The model under review builds one solid part; all positions refer to its coordinate system, in mm. Coordinates: 2 decimals unless noted, no trailing zeros. Order: outer loops, then holes, each group sorted by start corner. A loop starts at its lowest first (then second) coordinate and runs counter-clockwise, first axis right, second up.
from build123d import *

# Parameters (mm, degrees)
SKETCH_1_R      = 1.5
SKETCH_1_R_2    = 20
SKETCH_1_R_3    = 2.1
SKETCH_1_R_4    = 2
SKETCH_1_W      = 8.4
SKETCH_1_H      = 4.4
EXTRUDE_1_DEPTH = 4
EXTRUDE_2_DEPTH = 4
EXTRUDE_4_DEPTH = 4


with BuildPart() as part:
    # 草图1 → 凸台-拉伸1 (new body)
    with BuildSketch(Plane.XY):
        with BuildLine():
            Line((7.027428163, -5.002489357), (18.190287148, -14.686974418))
            ThreePointArc((18.190287148, -14.686974418), (47.018030055, -25.451404949), (75.84881126, -14.695114654))
            Line((75.84881126, -14.695114654), (87.027428163, -5.002489357))
            Line((87.027428163, -5.002489357), (87.027428163, 75.054738201))
            Line((87.027428163, 75.054738201), (21.027428163, 141.054738201))
            Line((21.027428163, 141.054738201), (-114.887663771, 141.054738201))
            ThreePointArc((-114.887663771, 141.054738201), (-124.126459096, 134.881572525), (-121.958731583, 123.983670389))
            Line((-121.958731583, 123.983670389), (-90.203942848, 92.228881654))
            Line((-90.203942848, 92.228881654), (7.027428163, -5.002489357))
        make_face()
        with Locations((-52.972571837, 135.054738201)):
            Circle(SKETCH_1_R, mode=Mode.SUBTRACT)
        with Locations((47.027428163, 15.054738201)):
            Circle(SKETCH_1_R_2, mode=Mode.SUBTRACT)
        with Locations(Location((-22.972571837, 135.054738201, 0), (0, 0, 180))):
            Circle(SKETCH_1_R, mode=Mode.SUBTRACT)
        with Locations((7.027428163, 135.054738201)):
            Circle(SKETCH_1_R, mode=Mode.SUBTRACT)
        with Locations(Location((-112.972571837, 135.054738201, 0), (0, 0, 180))):
            Circle(SKETCH_1_R, mode=Mode.SUBTRACT)
        with Locations((-82.972571837, 135.054738201)):
            Circle(SKETCH_1_R, mode=Mode.SUBTRACT)
        with Locations((49.784787476, 103.812097514)):
            Circle(SKETCH_1_R, mode=Mode.SUBTRACT)
        with Locations(Location((70.997990912, 82.598894078, 0), (0, 0, 180))):
            Circle(SKETCH_1_R, mode=Mode.SUBTRACT)
        with Locations(Location((28.571584041, 125.025300949, 0), (0, 0, 180))):
            Circle(SKETCH_1_R, mode=Mode.SUBTRACT)
        with Locations((70.597428163, 38.624738201)):
            Circle(SKETCH_1_R_3, mode=Mode.SUBTRACT)
        with Locations((70.597428163, -8.515261799)):
            Circle(SKETCH_1_R_3, mode=Mode.SUBTRACT)
        with Locations((23.457428163, -8.515261799)):
            Circle(SKETCH_1_R_3, mode=Mode.SUBTRACT)
        with Locations((23.457428163, 38.624738201)):
            Circle(SKETCH_1_R_3, mode=Mode.SUBTRACT)
        with Locations((-83.04451802, 93.554738201)):
            Circle(SKETCH_1_R, mode=Mode.SUBTRACT)
        with Locations((-61.831314585, 72.341534765)):
            Circle(SKETCH_1_R, mode=Mode.SUBTRACT)
        with Locations(Location((-104.257721456, 114.767941637, 0), (0, 0, 180))):
            Circle(SKETCH_1_R, mode=Mode.SUBTRACT)
        with Locations((20.166275086, 57.226748532)):
            Circle(SKETCH_1_R_4, mode=Mode.SUBTRACT)
        with Locations((-6.694877991, 99.398758863)):
            Circle(SKETCH_1_R_4, mode=Mode.SUBTRACT)
        with Locations((-37.972571837, 135.054738201)):
            Rectangle(SKETCH_1_W, SKETCH_1_H, mode=Mode.SUBTRACT)
        with Locations((-7.972571837, 135.054738201)):
            Rectangle(SKETCH_1_W, SKETCH_1_H, mode=Mode.SUBTRACT)
        with Locations((-97.972571837, 135.054738201)):
            Rectangle(SKETCH_1_W, SKETCH_1_H, mode=Mode.SUBTRACT)
        with Locations((-67.972571837, 135.054738201)):
            Rectangle(SKETCH_1_W, SKETCH_1_H, mode=Mode.SUBTRACT)
        Polygon((55.865905794, 94.619709358), (61.805602756, 88.680012396), (64.916872594, 91.791282234), (58.977175632, 97.730979196), align=None, mode=Mode.SUBTRACT)
        Polygon((34.652702359, 115.832912794), (37.763972196, 118.944182631), (43.703669158, 113.004485669), (40.592399321, 109.893215832), align=None, mode=Mode.SUBTRACT)
        Polygon((-73.852129865, 87.473619883), (-76.963399702, 84.362350046), (-71.02370274, 78.422653084), (-67.912432903, 81.533922921), align=None, mode=Mode.SUBTRACT)
        Polygon((-89.125636339, 102.747126356), (-92.236906176, 99.635856519), (-98.176603138, 105.575553481), (-95.065333301, 108.686823318), align=None, mode=Mode.SUBTRACT)
    extrude(amount=EXTRUDE_1_DEPTH)

    # 草图2 → 凸台-拉伸2 (add)
    with BuildSketch(Plane.XY.offset(4)):
        Polygon((87.027428163, -5.002489357), (87.027428163, -35.754116483), (67.811833288, -20.231246124), align=None)
    extrude(amount=-EXTRUDE_2_DEPTH)

    # 草图3 → 凸台-拉伸4 (add)
    with BuildSketch(Plane.XY.offset(4)):
        Polygon((7.027428163, 141.054738201), (5.027428163, 141.054738201), (7.027428163, 163.054738201), (9.027428163, 141.054738201), align=None)
    extrude(amount=-EXTRUDE_4_DEPTH)


solid = part.part
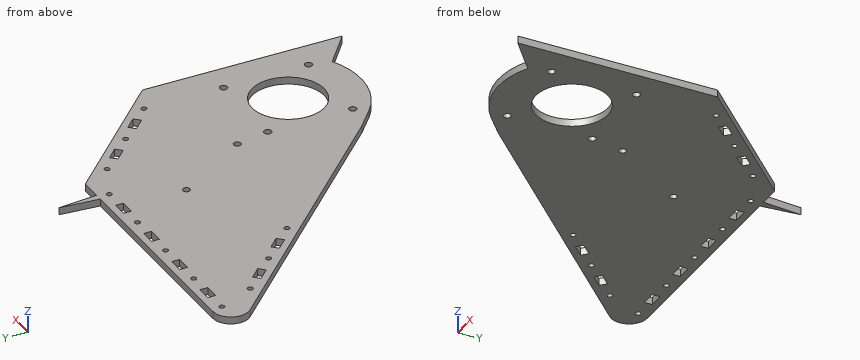
(1) Wall thickness on line 1 (Y direction, x = 58, z = 0.55); line 2 (Y direction, x = -33, z = 1.85); line 3 (X direction, y = 108, z = 3.45): over which ranges is each line inside the solid? List them lowest first.
(2) Consider section A-A (y = 31). Give the boundary of the cut face in (x, z), then the cut area to 3 significant figures.
(3) Consider section D-D (y = 65). Give the boundary of the cut face in (x, z), then the cut area to 3 significant figures.
(4) Insertion check: pin 1 Ø2 at (y, z) = (42, 2.5) entering from -X; pin 2 Ø2.5 at (x, y) = (28.57, 125.03) entering from -Z; pin 3 Ø2 at (x, z) = (-69, 1) entering from +Y; pin 4 Ø1 at (y, z) = (-12, 2.5) entering from -X. Each pin has a flat end and moves straight along its axis. Give the tip position at first contact, or say it passes through.
(5) Consider section C-C (z = 3.3). Give the number of separate pieces and of enclosed holes in the cut face, then the cut area to 3 significant figures.
(6) Consider section B-B (x = -39). Give the boundary of the cut face in (y, z).
Findings:
1. line 1: y = -24.06 to -1.67, 31.78 to 92.49, 96.75 to 104.08
1. line 2: y = 35.02 to 141.05
1. line 3: x = -105.98 to -95.75, -94.38 to 54.08
2. outline: (-28.98, 0) - (34.95, 0) - (34.95, 4) - (-28.98, 4) - close; (59.1, 0) - (87.03, 0) - (87.03, 4) - (59.1, 4) - close
2. area: 367 mm2
3. outline: (-62.98, 0) - (87.03, 0) - (87.03, 4) - (-62.98, 4) - close
3. area: 600 mm2
4. pin 1: stops at x = -40.98
4. pin 2: passes through
4. pin 3: stops at y = 141.05
4. pin 4: stops at x = 14.52
5. separate pieces: 1
5. enclosed holes: 26
5. area: 19,800 mm2
6. outline: (41.02, 0) - (132.85, 0) - (132.85, 4) - (41.02, 4) - close; (137.25, 0) - (141.05, 0) - (141.05, 4) - (137.25, 4) - close
